The model under review builds one solid part; all positions refer to its coordinate system, in mm. Face numbers are marked on the shaded views. A direction names the side the tool comes from. Round coordinates to 2 decimals unless told otherwise and drop trailing zeros. Order: outer loops, then holes, each group sorted by start corner. A loop starts at its lowest first (then second) coordinate and runs counter-clockwise, first axis right, second up. Notation, with made-up numbers: M 2,-22.75 L 56,-22.75 A19 ccw 56,-10.75 Z; hole C -37,-1 d3. An arc over 180 degrees is marked long. Use a Markdown table: item, result. Add a question column.
1. Consider section D-D on z = -2.5. State the section outline as (x, y) points, then the cut area to 3 significant figures.
2. Insertion check: P1, Ø1.5, axis at y = 1, z = -1, coming from the +X side; P2, Ø1, axis at y = 1.5, z = -2.5, coming from the +X side. Each pin has a flat end and moves straight along its axis. Give the tip position at first contact, or say it passes through.
3. Consider section B-B on x = 6. State the section outline as (y, z) points, then the cut area to 3 significant figures.
4. Consider section A-A on z = -3.5. State the section outline as (x, y) points, then the cut area to 3 significant figures.
5. Consider section C-C on y = 1.6. State the section outline as (x, z) points.
6. To check wall thickness, follow probe 1 along Y at (x, z) = (5.25, -3.5); probe 2 along X at (y, z) = (0.5, -3.5); probe 3 along Y at (x, z) = (3, -2.5). State the ranges of each line that lie inside material, in increasing order.
7. For the marked faces 1 and 2, list the 3-axis set-ups (+Z, -Z, +X, -X, +Y, -Y) from which the entire face can be reached by the end or side of a thin tool; tool diameter is ignored.
8. The part is to be moulded in two halves that separate along X. For the marked faces 3, 4, 5 and 6, say which applies: +X half, -X half, draft (parallel to the pull), parting line (faces both ways), or undercut.
from build123d import *

# Parameters (mm, degrees)
SKETCH1_W           = 7
SKETCH1_H           = 7
BOSS_EXTRUDE1_DEPTH = 3
CUT_EXTRUDE1_DEPTH  = 7
CUT_EXTRUDE2_DEPTH  = 11
SKETCH4_R           = 1.8
CUT_EXTRUDE3_DEPTH  = 0.8
CUT_EXTRUDE4_DEPTH  = 0.4


with BuildPart() as part:
    # Sketch1 → Boss-Extrude1 (new body)
    with BuildSketch(Plane(origin=(0, 0, 0), x_dir=(1, 0, 0), z_dir=(0, 1, 0))):
        with Locations((3.5, 3.5)):
            Rectangle(SKETCH1_W, SKETCH1_H)
    extrude(amount=BOSS_EXTRUDE1_DEPTH)

    # Sketch2 → Cut-Extrude1 (cut)
    with BuildSketch(Plane.XY):
        Polygon((0, 0), (0.7, 3), (0, 3), align=None)
        Polygon((7, 0), (6.3, 3), (7, 3), align=None)
    extrude(amount=-CUT_EXTRUDE1_DEPTH, mode=Mode.SUBTRACT)

    # Sketch3 → Cut-Extrude2 (cut)
    with BuildSketch(Plane(origin=(0, 0, 0), x_dir=(0, 0, -1), z_dir=(1, 0, 0))):
        Polygon((0, 0), (0.7, 3), (0, 3), align=None)
        Polygon((7, 3), (6.3, 3), (7, 0), align=None)
    extrude(amount=CUT_EXTRUDE2_DEPTH, mode=Mode.SUBTRACT)

    # Sketch4 → Cut-Extrude3 (cut)
    with BuildSketch(Plane.XZ):
        with Locations(Location((3.5, -3.5, 0), (0, 0, 270))):
            Circle(SKETCH4_R)
    extrude(amount=-CUT_EXTRUDE3_DEPTH, mode=Mode.SUBTRACT)

    # Sketch5 → Cut-Extrude4 (cut)
    with BuildSketch(Plane(origin=(0, 3, 0), x_dir=(1, 0, 0), z_dir=(0, 1, 0))):
        Polygon((1.943645472, 1.759282352), (3.143264863, 3.613048377), (2.078260857, 5.259282352), (2.864919511, 5.259282352), (3.53659419, 4.220920973), (4.20826887, 5.259282352), (4.994927523, 5.259282352), (3.929923517, 3.613048377), (5.129542908, 1.759282352), (4.342884254, 1.759282352), (3.53659419, 3.005175781), (2.730304126, 1.759282352), align=None)
    extrude(amount=-CUT_EXTRUDE4_DEPTH, mode=Mode.SUBTRACT)


solid = part.part
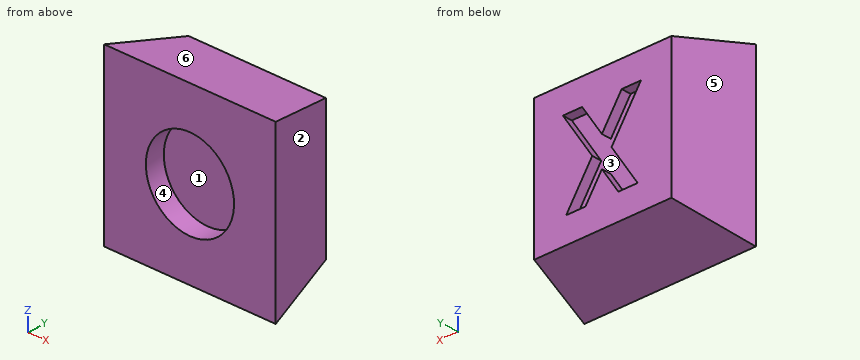
Answer block:
| question | item | result |
|---|---|---|
| 1 | outline | M 0,0 L 2,0 L 2,0.8 L 5,0.8 L 5,0 L 7,0 L 6.3,3 L 4.65,3 L 4.65,2.6 L 3.86,2.6 L 3.86,3 L 3.21,3 L 3.21,2.6 L 2.42,2.6 L 2.42,3 L 0.7,3 Z |
| 1 | area | 15.9 mm^2 |
| 2 | P1 | x = 6.94 |
| 2 | P2 | x = 6.77 |
| 3 | outline | M 0,-7 L 3,-6.3 L 3,-0.7 L 0,0 Z |
| 3 | area | 18.9 mm^2 |
| 4 | outline | M 0,0 L 1.7,0 L 1.7,0.8 L 5.3,0.8 L 5.3,0 L 7,0 L 6.3,3 L 4,3 L 4,2.6 L 3.07,2.6 L 3.07,3 L 0.7,3 Z |
| 4 | area | 15.6 mm^2 |
| 5 | outline | M 0.37,-6.63 L 6.63,-6.63 L 6.63,-0.37 L 0.37,-0.37 Z |
| 6 | probe 1 | 0.8 to 3 |
| 6 | probe 2 | 0.12 to 1.7, 5.3 to 6.88 |
| 6 | probe 3 | 0.8 to 2.6 |
| 7 | face 1 | -Y |
| 7 | face 2 | +Z, -Z, +X, +Y |
| 8 | face 3 | undercut |
| 8 | face 4 | undercut |
| 8 | face 5 | -X half |
| 8 | face 6 | draft |
